Check sheet for the modelled part. Datum: model origin and axes. Units: mm. A direction names the side the tool comes from. Coordinates: 2 decimals unless noted, no trailing zeros. Loops run counter-clockwise (first coordinate to the right, second up) from the corner with the lowest first, then second, coordinate; pieces in that order, holes last.
from build123d import *

# Parameters (mm, degrees)
EXTRUDE_1_DEPTH          = 14
SKETCH_3_R               = 13
CUT_EXTRUDE_1_DEPTH      = 423.251110123
PATTERN_LINEAR_1_COUNT   = 3
PATTERN_LINEAR_1_PITCH   = 80
MIRROR_1_COPY_1_SKETCH_R = 13
MIRROR_1_COPY_1_DEPTH    = 423.251110123
MIRROR_1_COPY_2_SKETCH_R = 13
MIRROR_1_COPY_2_DEPTH    = 423.251110123
EXTRUDE_2_DEPTH          = 12
SKETCH_7_R               = 13
CUT_EXTRUDE_2_DEPTH      = 423.819110259
SKETCH_8_W               = 500
SKETCH_8_H               = 12
EXTRUDE_5_DEPTH          = 78
SKETCH_9_R               = 13
CUT_EXTRUDE_3_DEPTH      = 435.644682471


with BuildPart() as part:
    # 草图1 → 凸台-拉伸1 (new body)
    with BuildSketch(Plane.XY):
        Polygon((0, 0), (250, 0), (250, 50), (100, 240), (100, 340), (0, 340), (-100, 340), (-100, 240), (-250, 50), (-250, 0), align=None)
    extrude(amount=EXTRUDE_1_DEPTH)

    # 草图3 → 切除-拉伸1 (cut, through all)
    with BuildSketch(Plane.XY.offset(14)):
        with Locations((-56, 290)):
            Circle(SKETCH_3_R)
    cut_extrude_1 = extrude(amount=-CUT_EXTRUDE_1_DEPTH, mode=Mode.SUBTRACT)

    # 阵列(线性)1: 切除-拉伸1 ×3
    with Locations(*[(0, -i * PATTERN_LINEAR_1_PITCH, 0) for i in range(1, PATTERN_LINEAR_1_COUNT)]):
        add(cut_extrude_1, mode=Mode.SUBTRACT)

    # 镜向1: 切除-拉伸1 across plane
    add(cut_extrude_1.mirror(Plane(origin=(0, 0, 0), x_dir=(0, 0, 1), z_dir=(1, 0, 0))), mode=Mode.SUBTRACT)

    # 镜向1 copy 1 sketch → 镜向1 copy 1 (cut, through all)
    with BuildSketch(Plane(origin=(0, -80, 14), x_dir=(-1, 0, 0), z_dir=(0, 0, 1))):
        with Locations((-56, -290)):
            Circle(MIRROR_1_COPY_1_SKETCH_R)
    extrude(amount=-MIRROR_1_COPY_1_DEPTH, mode=Mode.SUBTRACT)

    # 镜向1 copy 2 sketch → 镜向1 copy 2 (cut, through all)
    with BuildSketch(Plane(origin=(0, -160, 14), x_dir=(-1, 0, 0), z_dir=(0, 0, 1))):
        with Locations((-56, -290)):
            Circle(MIRROR_1_COPY_2_SKETCH_R)
    extrude(amount=-MIRROR_1_COPY_2_DEPTH, mode=Mode.SUBTRACT)

    # 草图6 → 凸台-拉伸2 (add)
    with BuildSketch(Plane.XY.offset(14)):
        Polygon((218.421052632, 90), (-218.421052632, 90), (-250, 50), (-250, 0), (250, 0), (250, 50), align=None)
    extrude(amount=EXTRUDE_2_DEPTH)

    # 草图7 → 切除-拉伸2 (cut, through all)
    with BuildSketch(Plane.XY.offset(26)):
        with Locations((-56, 50)):
            Circle(SKETCH_7_R)
        with Locations((-130, 50)):
            Circle(SKETCH_7_R)
        with Locations((-196, 50)):
            Circle(SKETCH_7_R)
    cut_extrude_2 = extrude(amount=-CUT_EXTRUDE_2_DEPTH, mode=Mode.SUBTRACT)

    # 镜向2: 切除-拉伸2 across plane
    add(cut_extrude_2.mirror(Plane(origin=(0, 0, 0), x_dir=(0, 0, 1), z_dir=(1, 0, 0))), mode=Mode.SUBTRACT)

    # 草图8 → 凸台-拉伸5 (add)
    with BuildSketch(Plane.XY.offset(26)):
        with Locations((0, 6)):
            Rectangle(SKETCH_8_W, SKETCH_8_H)
    extrude(amount=EXTRUDE_5_DEPTH)

    # 草图9 → 切除-拉伸3 (cut, through all)
    with BuildSketch(Plane.XZ):
        with Locations(Location((-180, 55, 0), (0, 0, 270))):
            Circle(SKETCH_9_R)
        with Locations(Location((-100, 55, 0), (0, 0, 270))):
            Circle(SKETCH_9_R)
    cut_extrude_3 = extrude(amount=-CUT_EXTRUDE_3_DEPTH, mode=Mode.SUBTRACT)

    # 镜向3: 切除-拉伸3 across plane
    add(cut_extrude_3.mirror(Plane(origin=(0, 0, 0), x_dir=(0, 0, 1), z_dir=(1, 0, 0))), mode=Mode.SUBTRACT)


solid = part.part
(1) Section check A-A, the plane y = 290. Enter the section's corners in (x, z).
(2) Section check B-B, the plane x = -130. Enter the section's corners in (y, z), plus the area to 3 significant figures.
(3) Gauge pin test, flat ends, axial feed: P1, Ø9.5, axis at x = 102, z = 21.5, coming from the +Y side; P2, Ø4, axis at x = -69, y = 252.5, coming from the +Z side; P3, Ø1, axis at x = 198, z = 91.5, coming from the +Y side. Record the tip position at first contact, or that the pin passes through.
(4) Section check C-C, the plane x = 56. Enter the section's corners in (y, z).
(5) Draft check along Z on faces 1 (the face through (-3, 6, 104)), 2 (the face through (100, 289, 7)), 3 (the face through (-192.69, 5.92, 57.82)). Enter one of: pulls with the +Z half, pulls with the -Z half, needs draft (parallel to the pull), parting line crosses it, or undercut.
(6) Section check D-D, the plane z = 21. Enter the section's corners in (x, y).
(7) Scan lines: line 1 along Y through (x, z) = (56, 11); line 2 along Y through (x, z) = (-56, 20.25); line 3 along Y through (x, z) = (-159.5, 46). Record each from-to range of solid material in increasing order.
(8) Set-up check for faces 4 (the face through (-107.91, 5.916, 65.316)), 5 (the face through (-3, 189, 14)), 6 (the face through (-100, 291, 7)): record each of +Z, -Z, +X, -X, +Y, -Y from which the full face is reachable in a straight line by a thin tool's end or side.
Determined:
1. outline: (-100, 0) - (-69, 0) - (-69, 14) - (-100, 14) - close; (-43, 0) - (43, 0) - (43, 14) - (-43, 14) - close; (69, 0) - (100, 0) - (100, 14) - (69, 14) - close
2. outline: (0, 0) - (37, 0) - (37, 26) - (12, 26) - (12, 104) - (0, 104) - close; (63, 0) - (202, 0) - (202, 14) - (90, 14) - (90, 26) - (63, 26) - close
2. area: 4,170 mm2
3. P1: stops at y = 90
3. P2: stops at z = 14
3. P3: stops at y = 12
4. outline: (0, 0) - (37, 0) - (37, 26) - (12, 26) - (12, 104) - (0, 104) - close; (63, 0) - (117, 0) - (117, 14) - (90, 14) - (90, 26) - (63, 26) - close; (143, 0) - (197, 0) - (197, 14) - (143, 14) - close; (223, 0) - (277, 0) - (277, 14) - (223, 14) - close; (303, 0) - (340, 0) - (340, 14) - (303, 14) - close
5. face 1: pulls with the +Z half
5. face 2: needs draft
5. face 3: undercut
6. outline: (-250, 0) - (250, 0) - (250, 50) - (218.42, 90) - (-218.42, 90) - (-250, 50) - close; hole circle Ø26 at (-196, 50); hole circle Ø26 at (-130, 50); hole circle Ø26 at (-56, 50); hole circle Ø26 at (56, 50); hole circle Ø26 at (130, 50); hole circle Ø26 at (196, 50)
7. line 1: y = 0 to 37, 63 to 117, 143 to 197, 223 to 277, 303 to 340
7. line 2: y = 0 to 37, 63 to 90
7. line 3: y = 0 to 12
8. face 4: +Y, -Y
8. face 5: +Z, +X, -X, +Y
8. face 6: +Z, -Z, -X, +Y
